from build123d import *

# Parameters (mm, degrees)
CROQUIS1_W              = 30
CROQUIS1_H              = 15
SALIENTE_EXTRUIR1_DEPTH = 5
CROQUIS2_W              = 30
CROQUIS2_H              = 5
SALIENTE_EXTRUIR2_DEPTH = 15
CROQUIS3_R              = 2
CORTAR_EXTRUIR1_DEPTH   = 15
CROQUIS4_R              = 0.5
CORTAR_EXTRUIR2_DEPTH   = 10


with BuildPart() as part:
    # Croquis1 → Saliente-Extruir1 (new body)
    with BuildSketch(Plane.XY):
        with Locations((15, 7.5)):
            Rectangle(CROQUIS1_W, CROQUIS1_H)
    extrude(amount=SALIENTE_EXTRUIR1_DEPTH)

    # Croquis2 → Saliente-Extruir2 (add)
    with BuildSketch(Plane.XY.offset(5)):
        with Locations((15, 12.5)):
            Rectangle(CROQUIS2_W, CROQUIS2_H)
    extrude(amount=SALIENTE_EXTRUIR2_DEPTH)

    # Croquis3 → Cortar-Extruir1 (cut)
    with BuildSketch(Plane.XY.offset(5)):
        with Locations((24, 5)):
            Circle(CROQUIS3_R)
        with Locations((6, 5)):
            Circle(CROQUIS3_R)
    extrude(amount=-CORTAR_EXTRUIR1_DEPTH, mode=Mode.SUBTRACT)

    # Croquis4 → Cortar-Extruir2 (cut)
    with BuildSketch(Plane(origin=(0, 10, 0), x_dir=(-1, 0, 0), z_dir=(0, -1, 0))):
        with Locations((-15, -11)):
            Circle(CROQUIS4_R)
    extrude(amount=-CORTAR_EXTRUIR2_DEPTH, mode=Mode.SUBTRACT)


solid = part.part
Check sheet for the modelled part. Datum: model origin and axes. Units: mm. A direction names the side the tool comes from. Round coordinates to 2 decimals unless told otherwise and drop trailing zeros. Loops run counter-clockwise (first coordinate to the right, second up) from the corner with the lowest first, then second, coordinate; pieces in that order, holes last.
1. Scan lines: probe 1 along Y at (x, z) = (24, 2.2); probe 2 along Y at (x, z) = (5, 16); probe 3 along Z at (x, y) = (1.5, 4.25). Record each from-to range of solid material in increasing order.
2. Sectioned sample at B-B on x = 6. Record the boundary of the cut face in (y, z), and give its area (3 significant figures).
3. Sectioned sample at D-D on x = 15. Record the boundary of the cut face in (y, z).
4. Mould release check, pull along Y, two halves, no side actions. Record for faces 3 (the cylindrical face through (4, 5, 3)), 4 (the cylindrical face through (22, 5, 3)), 5 (the flat face through (15, 13, 20)), 6 (the flat face through (15, 0, 2)): released by +Y, released by -Y, zero draft, split by the parting line, or undercut.
5. Gauge pin test, flat ends, axial feed: pin 1 Ø6.5 at (x, y) = (24, 5) entering from +Z; pin 2 Ø2.5 at (x, y) = (6, 5) entering from -Z. Record the tip position at first contact, or that the pin passes through.
6. Sectioned sample at A-A on z = 11. Record the boundary of the cut face in (x, y).
7. Sectioned sample at C-C on y = 5. Record the boundary of the cut face in (x, z).
8. Set-up check for faces 1 (the cylindrical face through (14.769, 12.465, 11.444)), 2 (the flat face through (15, 5, 5)): record each of +Z, -Z, +X, -X, +Y, -Y from which the full face is reachable in a straight line by a thin tool's end or side.
Recorded:
1. probe 1: y = 0 to 3, 7 to 15
1. probe 2: y = 10 to 15
1. probe 3: z = 0 to 5
2. outline: (0, 0) - (3, 0) - (3, 5) - (0, 5) - close; (7, 0) - (15, 0) - (15, 20) - (10, 20) - (10, 5) - (7, 5) - close
2. area: 130 mm2
3. outline: (0, 0) - (15, 0) - (15, 10.5) - (10, 10.5) - (10, 5) - (0, 5) - close; (10, 11.5) - (15, 11.5) - (15, 20) - (10, 20) - close
4. face 3: undercut
4. face 4: undercut
4. face 5: zero draft
4. face 6: released by -Y
5. pin 1: stops at z = 5
5. pin 2: passes through
6. outline: (0, 10) - (14.5, 10) - (14.5, 15) - (0, 15) - close; (15.5, 10) - (30, 10) - (30, 15) - (15.5, 15) - close
7. outline: (0, 0) - (4, 0) - (4, 5) - (0, 5) - close; (8, 0) - (22, 0) - (22, 5) - (8, 5) - close; (26, 0) - (30, 0) - (30, 5) - (26, 5) - close
8. face 1: +Y, -Y
8. face 2: +Z, +X, -X, -Y
